from build123d import *

# Parameters (mm, degrees)
F0_R     = 57.15
F0_R_2   = 25.4
F1_DEPTH = 25.4
F0_R_3   = 76.2
F2_DEPTH = 1.5875
F3_DEPTH = 53.975
F4_R     = 4.7625
F5_DEPTH = 3.176


with BuildPart() as f1:
    # F0 (on Front) → F1 (new body)
    with BuildSketch(Plane.XZ):
        Circle(F0_R)
        Circle(F0_R_2, mode=Mode.SUBTRACT)
    extrude(amount=F1_DEPTH)

    # F0 (on Front) → F2 (join, symmetric)
    with BuildSketch(Plane.XZ):
        Circle(F0_R_3)
        Circle(F0_R, mode=Mode.SUBTRACT)
    extrude(amount=F2_DEPTH, both=True)

    # F0 (on Front) → F3 (join)
    with BuildSketch(Plane.XZ):
        Circle(F0_R_2)
    extrude(amount=F3_DEPTH)

    # F4 (on face) → F5 (cut, through all)
    with BuildSketch(Plane.XZ.offset(1.5875)):
        with Locations((61.95407, -25.41648)):
            Circle(F4_R)
    extrude(amount=-F5_DEPTH, mode=Mode.SUBTRACT)


solid = f1.part
Input: part model. Units: mm. Frame: model coordinates. A direction names the side the tool comes from. Coordinates: 2 decimals unless noted, no trailing zeros. Loops run counter-clockwise (first coordinate to the right, second up) from the corner with the lowest first, then second, coordinate; pieces in that order, holes last.
(1) First-contact query: pin 1 Ø1.5 at (x, z) = (60.5, 35.5) entering from -Y; pin 2 Ø12 at (x, y) = (-13.5, -31.5) entering from +Z; pin 3 Ø1 at (x, z) = (45, -23) entering from -Y. Flat tips, straight axial feed; report the tip coordinate or a pass-through.
(2) Section C-C on y = -11. Return the cut outline in (x, z).
(3) Pull-direction query (Z, two-part tool) for faces 4 (the face through (28, -1.588, -50)), 5 (the face through (-5.506, -39.487, -24.796)), 6 (the face through (66.5, 0, -24)); classes: released by +Z, released by -Z, zero draft, split by the parting line, or undercut.
(4) Section D-D on x = 38.5. Return the cut outline in (y, z).
(5) Material intervals for probe 1 along Z at (x, y) = (0, 0.3); probe 2 along Y at (x, z) = (5.5, 14) (3 decimals); probe 3 along Y at (x, z) = (-10.5, -51.5), sorted ascending.
(6) Set-up query: faces 1 (the face through (28, 1.588, -50)), 2 (the face through (-1, 0, 1)), 3 (the face through (25, -25.4, -12)). Return all of +Z, -Z, +X, -X, +Y, -Y with unobstructed straight access to the full face (end or side cutting, diameter ignored); none if empty.
Data:
1. pin 1: stops at y = -1.59
1. pin 2: stops at z = 24.27
1. pin 3: stops at y = -25.4
2. outline: circle Ø114.3 at (0, 0)
3. face 4: zero draft
3. face 5: split by the parting line
3. face 6: undercut
4. outline: (-25.4, -42.24) - (-1.59, -42.24) - (-1.59, -65.76) - (1.59, -65.76) - (1.59, -42.24) - (0, -42.24) - (0, 42.24) - (1.59, 42.24) - (1.59, 65.76) - (-1.59, 65.76) - (-1.59, 42.24) - (-25.4, 42.24) - close
5. probe 1: z = -76.2 to -57.15, 57.15 to 76.2
5. probe 2: y = -53.975 to 0
5. probe 3: y = -25.4 to 0
6. face 1: +Z, -Z, +X, -X, +Y
6. face 2: +Y
6. face 3: -Y
